Autodesk Inventor part; units mm, degrees
ref_plane "YZ Plane" through (0, 0, 0) normal (1, 0, 0) x (0, 1, 0)
ref_plane "XZ Plane" through (0, 0, 0) normal (0, 1, 0) x (-1, 0, 0)
ref_plane "XY Plane" through (0, 0, 0) normal (0, 0, 1) x (1, 0, 0)
sketch "Sketch1" plane through (0, 0, 0) normal (0, 0, 1) x (1, 0, 0)
  line L0 (-25, 0) -> (25, 0)
  line L1 (25, 0) -> (25, -860)
  line L2 (25, -860) -> (-25, -860)
  line L3 (-25, -860) -> (-25, 0)
  line L4 (25, 0) -> (-25, -68.0668)
  point P0 (0, 0)
  point P1 (0, 0)
  point P2 (25, -1153.2713)
  dimension "d0" = 50
  dimension "d1" = 860
  dimension "d6" = 53.7
extrude "Plate1" add sketch "Sketch1" along normal mid plane 3 contours L1 L2 L3 L4
chamfer "Corner Chamfer2" distance 3 angle 45 1 edges at (25, 0, 0)
fillet "Corner Round1" radius 6 1 edges at (-25, -68.0668, 0)
sketch "Sketch2" plane through (0, 0, 1.5) normal (0, 0, 1) x (1, 0, 0)
  line L0 (25, -186.5) -> (-1, -186.5)
  line L1 (-1, -186.5) -> (-1, -189.5)
  line L2 (-1, -189.5) -> (25, -189.5)
  line L3 (25, -189.5) -> (25, -186.5)
  line L4 (25, -3) -> (25, -860)
  point P0 (0, 0)
  point P1 (25, -188)
  point P2 (25, -827)
  dimension "d15" = 188
  dimension "d16" = 26
  dimension "d17" = 3
extrude "Extrusion1" cut sketch "Sketch2" against normal through all
pattern_linear "Rectangular Pattern1" count 3 spacing 323 along (0, -1, 0) of "Extrusion1"
fillet "Corner Round3" radius 6 1 edges at (-25, -860, 0)
sketch "Sketch3" plane through (0, 0, -1.5) normal (0, 0, -1) x (-1, 0, 0)
  line L0 (-4.7159, -271.7572) -> (4.3119, -271.7572) construction
  line L1 (4.3119, -271.7572) -> (4.3119, -401.2704) construction
  line L2 (4.3119, -401.2704) -> (-4.7159, -401.2704) construction
  line L3 (-4.7159, -401.2704) -> (-4.7159, -271.7572) construction
  point P0 (0, 0)
mark "Mark1"
equation "\"d6\" = d5"
equation "\"d2\" = Thickness"
equation "\"BendReliefWidth\" = Thickness"
equation "\"BendReliefDepth\" = 0.5 * Thickness"
equation "\"CornerReliefSize\" = 4 * Thickness"
equation "\"MinimumRemnant\" = 2 * Thickness"
equation "\"TransitionRadius\" = BendRadius"
equation "\"JacobiRadiusSize\" = BendRadius"
equation "\"GapSize\" = Thickness"
properties part number "MSC 603 STRINGER CONE EXIT BACK" material "Stainless Steel"
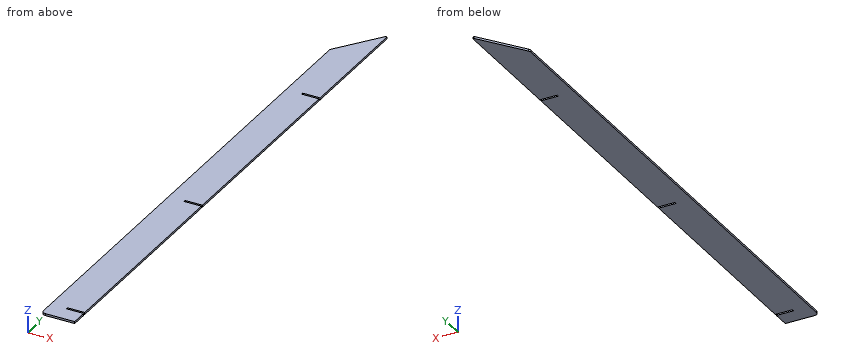
Could you check a few things on this model? Use its own coordinates, in mm. Coordinates: 2 decimals unless noted, no trailing zeros. Order: outer loops, then holes, each group sorted by start corner. A loop starts at its lowest first (then second) coordinate and runs counter-clockwise, first axis right, second up. Notation, with made-up numbers: (-20, 82) -> (6, 82) arc R25 cw to (6, 109) -> close; hole circle Ø6 at (52.25, 9.5). An arc over 180 degrees is marked (long way). One line per question, with ' | ' between items.
Q1. I'm going to push flat-ended pins straight in: P1, Ø0.9, axis at x = 8, z = -0.5, coming from the +Y side; P2, Ø1.5, axis at y = -510.5, z = 0.5, coming from the +X side; P3, Ø0.9, axis at x = 12.5, z = -0.5, coming from the +Y side. Where does each tip first touch, or does it pass through?
Return value:
P1: y = -22.53 | P2: x = -1 | P3: y = -16.4
Q2. Imagine slicing it at B-B on x = 9. Please give me the cut outline in (y, z), and give its area (3 significant figures).
Return value:
outline: (-860, -1.5) -> (-835.5, -1.5) -> (-835.5, 1.5) -> (-860, 1.5) -> close; (-832.5, -1.5) -> (-512.5, -1.5) -> (-512.5, 1.5) -> (-832.5, 1.5) -> close; (-509.5, -1.5) -> (-189.5, -1.5) -> (-189.5, 1.5) -> (-509.5, 1.5) -> close; (-186.5, -1.5) -> (-21.78, -1.5) -> (-21.78, 1.5) -> (-186.5, 1.5) -> close | area: 2,490 mm²
Q3. If I drill on L1, parallel to Y at x = -0.5, z = -1.2; L2, parallel to Y at x = 12.5, z = 0.2; L3, parallel to Y at x = -10.5, z = 0.7, over which ranges is the centre line in solid material (lowest first)?
Return value:
L1: -860 to -835.5, -832.5 to -512.5, -509.5 to -189.5, -186.5 to -34.71 | L2: -860 to -835.5, -832.5 to -512.5, -509.5 to -189.5, -186.5 to -17.02 | L3: -860 to -48.33
Q4. Imagine slicing it at A-A on z = -0.4. Please give me the cut outline in (x, y).
Return value:
outline: (-25, -854) arc R6 ccw to (-19, -860) -> (25, -860) -> (25, -835.5) -> (-1, -835.5) -> (-1, -832.5) -> (25, -832.5) -> (25, -512.5) -> (-1, -512.5) -> (-1, -509.5) -> (25, -509.5) -> (25, -189.5) -> (-1, -189.5) -> (-1, -186.5) -> (25, -186.5) -> (25, -3) -> (23.22, -2.42) -> (-23.84, -66.48) arc R6 ccw to (-25, -70.03) -> close
